```python
from build123d import *


with BuildPart() as f1:
    # F0 (on Front) → F1 (revolve)
    with BuildSketch(Plane.XZ):
        Polygon((-2.5, 0), (0, 0), (0, 5), (-3, 5), (-3, 4.5), (-2.5, 4.5), align=None)
        with BuildLine():
            Line((-3, 5), (0, 5))
            Line((0, 5), (0, 6))
            ThreePointArc((0, 6), (-1.581139, 5.743416), (-3, 5))
        make_face()
    revolve(axis=Axis((0, 0, 2.5), (0, 0, 1)))

    # F2: F1 across face


with BuildPart() as f1_1:
    add(f1.part)
    add(f1.part.mirror(Plane(origin=(0, 0, 0), x_dir=(1, 0, 0), z_dir=(0, 0, -1))))


solid = f1_1.part
```
Could you check a few things on this model? Use its own coordinates, in mm. A direction names the side the tool comes from. Round coordinates to 2 decimals unless told otherwise and drop trailing zeros. Loops run counter-clockwise (first coordinate to the right, second up) from the corner with the lowest first, then second, coordinate; pieces in that order, holes last. Notation, with made-up numbers: (58, 42) - (102, 42) arc R8 ccw to (102, 54) - close; hole circle Ø8 at (-2, -2). An arc over 180 degrees is marked (long way). Answer in a Markdown table with one row per item. Add a question column.
(1) If we mould it in two halves opening along Z, with no side actions, what happens to faces 3 (the face through (2, -2, -4.5)), 4 (the face through (3, -0.1, 4.7)), 5 (the face through (0.54, 2.44, 0.06))? For each: pulls with the +Z half, pulls with the -Z half, needs draft (parallel to the pull), parting line crosses it, or undercut.
(2) I need wall thicknesses on line 1 along Z through (x, y) = (-1.5, -2.25); line 2 along Y through (x, z) = (0, 3.5). Which ranges of each line are inside material? Lowest first, please.
(3) I'm going to push flat-ended pins straight in: pin 1 (1.5 mm diameter, centred on x = 1, y = 2, fed in from -Z); pin 2 (1 mm diameter, centred on x = -1.5, y = 2, fed in from +Z); pin 3 (3 mm diameter, centred on y = 1.5, z = 2.5, fed in from -X). Where does each tip first touch, or does it pass through?
(4) For faces 1 (the face through (3, -0.1, -4.7)), 2 (the face through (2, -2, 4.5)), which set-ups out of +Z, -Z, +X, -X, +Y, -Y let a thin tool reach every point of the face, with its end or its side?
(5) If we section it at A-A (z = 4): Please give me the cut outline in (x, y).
Model answer:
| question | item | result |
|---|---|---|
| 1 | face 3 | undercut |
| 1 | face 4 | needs draft |
| 1 | face 5 | undercut |
| 2 | line 1 | z = -5.21 to -4.5, 4.5 to 5.21 |
| 2 | line 2 | y = -2.5 to 2.5 |
| 3 | pin 1 | stops at z = -5.77 |
| 3 | pin 2 | stops at z = 5.58 |
| 3 | pin 3 | stops at x = -2.5 |
| 4 | face 1 | +Z, -Z |
| 4 | face 2 | none |
| 5 | outline | circle Ø5 at (0, 0) |
